Design review of the part built by this model. Coordinates are the model's own, in mm. Face numbers are marked on the shaded views. A direction names the side the tool comes from. Give positions to 0.01 mm unless a question says otherwise; leave off trailing zeros. Order: outer loops, then holes, each group sorted by start corner. A loop starts at its lowest first (then second) coordinate and runs counter-clockwise, first axis right, second up. Notation, with made-up numbers: (82, 31.5) -> (102, 31.5) arc R23 cw to (102, 56.5) -> close; hole circle Ø2 at (-23, 57.5). An arc over 180 degrees is marked (long way). Answer in a Markdown table with one row per item. Add a question column.
```python
from build123d import *

# Parameters (mm, degrees)
SKETCH2_W           = 20
SKETCH2_H           = 10
SKETCH2_R           = 2.5
BOSS_EXTRUDE1_DEPTH = 5
SKETCH2_3_W         = 20
SKETCH2_3_H         = 10
BOSS_EXTRUDE2_DEPTH = 25
SKETCH4_R           = 4.25
CUT_EXTRUDE1_DEPTH  = 88
SKETCH5_R           = 1.5
CUT_EXTRUDE2_DEPTH  = 88
FILLET1_R           = 5
FILLET2_R           = 2


with BuildPart() as part:
    # Sketch2 → Boss-Extrude1 (new body)
    # profile 1 of 2: a face of its own
    with BuildSketch(Plane(origin=(0, 0, 0), x_dir=(1, 0, 0), z_dir=(0, 1, 0))):
        with Locations((0, -5)):
            Rectangle(SKETCH2_W, SKETCH2_H)
        with Locations(Location((0, -6.5, 0), (0, 0, 270))):
            Circle(SKETCH2_R, mode=Mode.SUBTRACT)
    # profile 2 of 2: a face of its own
    with BuildSketch(Plane(origin=(0, 0, 0), x_dir=(1, 0, 0), z_dir=(0, 1, 0))):
        with Locations((0, 5)):
            Rectangle(SKETCH2_W, SKETCH2_H)
    extrude(amount=BOSS_EXTRUDE1_DEPTH)

    # Sketch2_3 → Boss-Extrude2 (add)
    with BuildSketch(Plane(origin=(0, 0, 0), x_dir=(1, 0, 0), z_dir=(0, 1, 0))):
        with Locations((0, 5)):
            Rectangle(SKETCH2_3_W, SKETCH2_3_H)
    extrude(amount=BOSS_EXTRUDE2_DEPTH)

    # Sketch4 → Cut-Extrude1 (cut)
    with BuildSketch(Plane.XY):
        with Locations((0, 15)):
            Circle(SKETCH4_R)
    extrude(amount=-CUT_EXTRUDE1_DEPTH, mode=Mode.SUBTRACT)

    # Sketch5 → Cut-Extrude2 (cut)
    with BuildSketch(Plane(origin=(10, 0, 0), x_dir=(0, 0, -1), z_dir=(1, 0, 0))):
        with Locations((5, 15)):
            Circle(SKETCH5_R)
    extrude(amount=-CUT_EXTRUDE2_DEPTH, mode=Mode.SUBTRACT)

    # Fillet1
    fillet1_edges = [part.edges().sort_by_distance(p)[0] for p in [
        (-10, 25, -5),
        (10, 25, -5),
    ]]
    fillet(fillet1_edges, radius=FILLET1_R)

    # Fillet2
    fillet2_edges = [part.edges().sort_by_distance(p)[0] for p in [
        (0, 5, 0),
    ]]
    fillet(fillet2_edges, radius=FILLET2_R)


solid = part.part
```
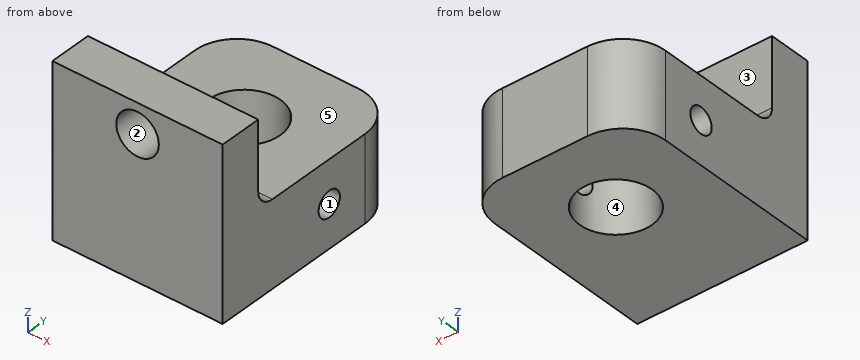
1) Add section D-D, the plane z = -1.75. Write out the cut boundary in (x, y).
2) Mouldability with a two-part tool opening along Y and no side actions: class the marked faces 1, 2 and 3 as +Y half, -Y half, draft (parallel to the pull), parting line (faces both ways), or undercut.
3) Machinability: for the marked faces 4 and 5, which of the approach directions +Z, -Z, +X, -X, +Y, -Y give a long, thin tool a straight path to every point of the face, cutting with its end or side? Answer none if there is none.
4) Add section C-C, the plane y = 15. Write out the cut boundary in (x, z).
5) For L1, parallel to X at y = 2.8, z = 6.5; L2, parallel to Z at x = -8, y = 15; L3, parallel to Y at x = -7, z = 3, list the stretches that pass through material, from the lowest coordinate up.
6) Add section A-A, the plane z = 6.5. Write out the cut boundary in (x, y), and give its area (3 significant figures).
7) Clearance check with a flat-ended pin moving along its axis: P1, Ø4, axis at x = -3.5, z = 4.5, coming from the +Y side. State where the tip first meets the part, or that it passes through.
8) Add section B-B, the plane x = 0. Write out the cut boundary in (y, z).
Verdict:
| question | item | result |
|---|---|---|
| 1 | outline | (-10, 0) -> (10, 0) -> (10, 20) arc R5 ccw to (5, 25) -> (-5, 25) arc R5 ccw to (-10, 20) -> close; hole circle Ø8.5 at (0, 15) |
| 2 | face 1 | undercut |
| 2 | face 2 | draft |
| 2 | face 3 | +Y half |
| 3 | face 4 | +Z, -Z |
| 3 | face 5 | +Z, +X, -X, +Y |
| 4 | outline | (-10, -10) -> (-4.25, -10) -> (-4.25, -6.5) -> (-10, -6.5) -> close; (-10, -3.5) -> (-4.25, -3.5) -> (-4.25, 0) -> (-10, 0) -> close; (4.25, -10) -> (10, -10) -> (10, -6.5) -> (4.25, -6.5) -> close; (4.25, -3.5) -> (10, -3.5) -> (10, 0) -> (4.25, 0) -> close |
| 5 | L1 | x = -10 to -2.5, 2.5 to 10 |
| 5 | L2 | z = -10 to -6.5, -3.5 to 0 |
| 5 | L3 | y = 0 to 5 |
| 6 | outline | (-10, 0) -> (-2.5, 0) -> (-2.5, 5) -> (-10, 5) -> close; (2.5, 0) -> (10, 0) -> (10, 5) -> (2.5, 5) -> close |
| 6 | area | 75.0 mm2 |
| 7 | P1 | stops at y = 5 |
| 8 | outline | (0, -10) -> (10.75, -10) -> (10.75, 0) -> (7, 0) arc R2 cw to (5, 2) -> (5, 4) -> (0, 4) -> close; (0, 9) -> (5, 9) -> (5, 10) -> (0, 10) -> close; (19.25, -10) -> (25, -10) -> (25, 0) -> (19.25, 0) -> close |
